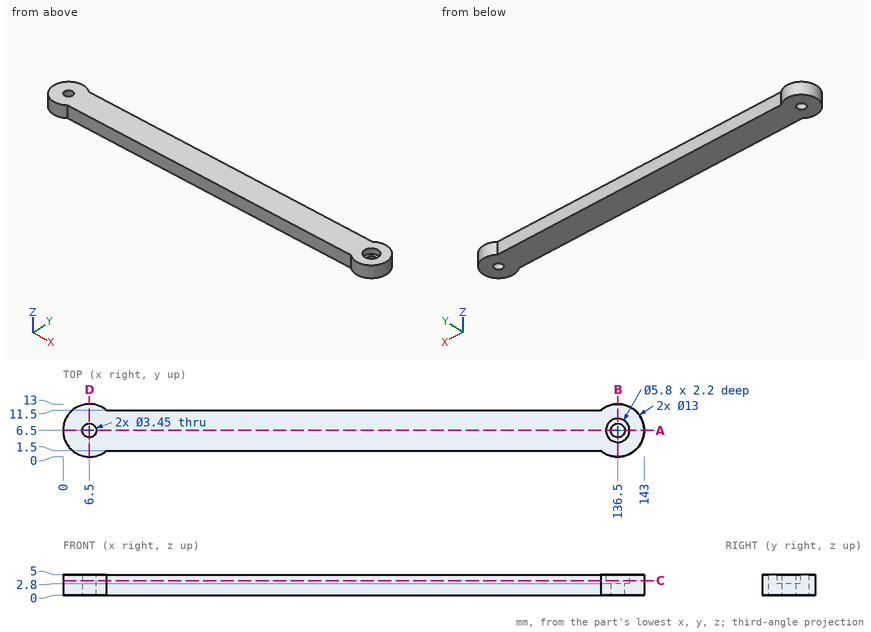
The drawing under review shows one solid part. Ordinate dimensions are in mm from its lowest x, y, z. Give positions to 0.01 mm unless a question says otherwise; leave off trailing zeros. Write each loop counter-clockwise with the first axis right and the second up, starting at its lowest first coordinate (ties: lowest second). Pieces come first, ordered by that corner, then holes. Notation, with made-up numbers: (2.5, -38.75) -> (57.5, -38.75) arc R22 ccw to (57.5, -29.75) -> close; hole circle Ø8 at (25.5, 56.25). An arc over 180 degrees is marked (long way). Put each result on its own line as item: value.
(1) We need section D-D, the plane x = 6.5. Give the boundary of the cut face in (y, z) (3 decimals).
Results are:
outline: (0, 0) -> (4.775, 0) -> (4.775, 5) -> (0, 5) -> close; (8.225, 0) -> (13, 0) -> (13, 5) -> (8.225, 5) -> close
(2) To check wall thickness, follow probe 1 along Y at (x, z) = (136.5, 3.7); probe 2 along X at (y, z) = (6.75, 4.1); probe 3 along X at (y, z) = (5, 1.05). State the ranges of each line that lie inside material, in increasing order. Write a range as from..to.
Results are:
probe 1: 0..3.6, 9.4..13
probe 2: 0..4.79, 8.21..133.61, 139.39..143
probe 3: 0.18..5.65, 7.35..135.65, 137.35..142.82
(3) We need section A-A, the plane y = 6.5. Give the boundary of the cut face in (x, z) (3 decimals), and give its area (3 significant figures).
Results are:
outline: (0, 0) -> (4.775, 0) -> (4.775, 5) -> (0, 5) -> close; (8.225, 0) -> (134.775, 0) -> (134.775, 2.8) -> (133.6, 2.8) -> (133.6, 5) -> (8.225, 5) -> close; (138.225, 0) -> (143, 0) -> (143, 5) -> (139.4, 5) -> (139.4, 2.8) -> (138.225, 2.8) -> close
area: 675 mm²
(4) We need section B-B, the plane x = 136.5. Give the boundary of the cut face in (y, z) (3 decimals), and give its area (3 significant figures).
Results are:
outline: (0, 0) -> (4.775, 0) -> (4.775, 2.8) -> (3.6, 2.8) -> (3.6, 5) -> (0, 5) -> close; (8.225, 0) -> (13, 0) -> (13, 5) -> (9.4, 5) -> (9.4, 2.8) -> (8.225, 2.8) -> close
area: 42.6 mm²
(5) For pin 1 Ø2 at (x, y) = (6.5, 6.5) entering from +Z; pin 2 Ø1 at (y, z) = (2.5, 3.5) entering from +X; pin 3 Ø2 at (x, z) = (22, 1) entering from +Y, all flat-tipped, find the tip position at first contact; note any pin that passes through.
Results are:
pin 1: through
pin 2: x = 141.98
pin 3: y = 11.5
(6) We need section C-C, the plane z = 3.6. Give the boundary of the cut face in (x, y) (3 decimals), and give its area (3 significant figures).
Results are:
outline: (10.653, 1.5) -> (132.347, 1.5) arc R6.5 ccw (long way) to (132.347, 11.5) -> (10.653, 11.5) arc R6.5 ccw (long way) to start; hole circle Ø3.45 at (6.5, 6.5); hole circle Ø5.8 at (136.5, 6.5)
area: 1,410 mm²
